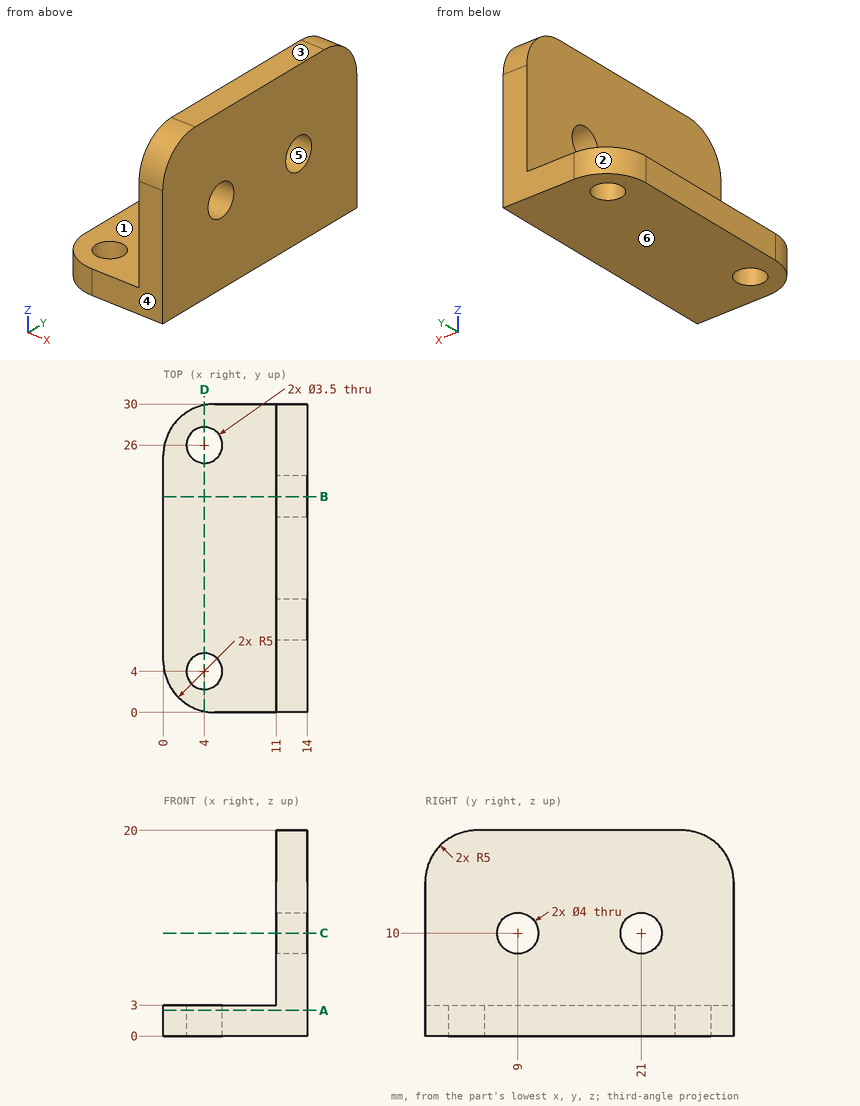
The figure shows three views and two pictorial views of one solid part (mm, origin at its lowest corner). Answer the questions. A direction names the side the tool comes from. Give positions to 0.01 mm unless a question says otherwise; leave off trailing zeros. Write each loop counter-clockwise with the first axis right and the second up, starting at its lowest first coordinate (ties: lowest second). Pieces come first, ordered by that corner, then holes. Notation, with made-up numbers: (-24.5, -8.75) - (-19.5, -8.75) arc R21 ccw to (-19.5, 19.25) - close; hole circle Ø5 at (11, -38.5). An arc over 180 degrees is marked (long way). Return JSON: item names as keys, results as strings.
Q1. A cutting plane is placed at D-D, the plane x = 4. Determine the outline of the cut face in (y, z).
Reply:
{"outline": "(0.1, 0) - (2.25, 0) - (2.25, 3) - (0.1, 3) - close; (5.75, 0) - (24.25, 0) - (24.25, 3) - (5.75, 3) - close; (27.75, 0) - (29.9, 0) - (29.9, 3) - (27.75, 3) - close"}
Q2. For the marked faces 1 and 2, determine the directions among +Z, -Z, +X, -X, +Y, -Y from which every point of the face is accessible in a straight line to the end or side of a thin tool.
Reply:
{"face 1": "+Z, -X, +Y, -Y", "face 2": "+Z, -Z, -X, +Y"}
Q3. Given P1, Ø3, axis at y = 21, z = 10, coming from the +X side; P2, Ø5, axis at y = 10, z = 14, coming from the -X side, each flat-ended and moving along its own axis, determine where each tip first touches the part or whether it passes through.
Reply:
{"P1": "through", "P2": "x = 11"}
Q4. A cutting plane is placed at A-A, the plane z = 2.5. Determine the outline of the cut face in (x, y), and give its area (3 significant figures).
Reply:
{"outline": "(0, 5) arc R5 ccw to (5, 0) - (14, 0) - (14, 30) - (5, 30) arc R5 ccw to (0, 25) - close; hole circle Ø3.5 at (4, 4); hole circle Ø3.5 at (4, 26)", "area": "390 mm²"}
Q5. A cutting plane is placed at B-B, the plane y = 21. Determine the outline of the cut face in (x, z), and give its area (3 significant figures).
Reply:
{"outline": "(0, 0) - (14, 0) - (14, 8) - (11, 8) - (11, 3) - (0, 3) - close; (11, 12) - (14, 12) - (14, 20) - (11, 20) - close", "area": "81.0 mm²"}
Q6. For a pull along Z with two mould halves and no side action, classify the marked faces 3, 4, 5 and 6 as released by +Z, released by -Z, zero draft, split by the parting line, or undercut.
Reply:
{"face 3": "released by +Z", "face 4": "zero draft", "face 5": "undercut", "face 6": "released by -Z"}
Q7. A cutting plane is placed at C-C, the plane z = 10. Determine the outline of the cut face in (x, y).
Reply:
{"outline": "(11, 0) - (14, 0) - (14, 7) - (11, 7) - close; (11, 11) - (14, 11) - (14, 19) - (11, 19) - close; (11, 23) - (14, 23) - (14, 30) - (11, 30) - close"}
Q8. Consider line 1 along Y through (x, z) = (12.45, 10); line 2 along Y through (x, z) = (4, 2.45); line 3 along Z through (x, y) = (6.75, 10). Determine where each line is inside the solid, lowest interval first. Write a range as [from, to].
Reply:
{"line 1": "[0, 7], [11, 19], [23, 30]", "line 2": "[0.1, 2.25], [5.75, 24.25], [27.75, 29.9]", "line 3": "[0, 3]"}
